```python
from build123d import *

# Parameters (mm, degrees)
BOSS_EXTRUDE1_DEPTH = 1
SKETCH2_W           = 3
SKETCH2_H           = 2.1
SKETCH2_W_2         = 1.6
SKETCH2_H_2         = 0.5
BOSS_EXTRUDE2_DEPTH = 0.1


with BuildPart() as part:
    # Sketch1 → Boss-Extrude1 (new body)
    with BuildSketch(Plane(origin=(0, 0, 0), x_dir=(1, 0, 0), z_dir=(0, 1, 0))):
        with BuildLine():
            Line((-10, 6.5), (10, 6.5))
            Line((10, 6.5), (10, 1))
            Line((10, 1), (9.1, 1))
            ThreePointArc((9.1, 1), (8.1, 0), (9.1, -1))
            Line((9.1, -1), (10, -1))
            Line((10, -1), (10, -6.5))
            Line((10, -6.5), (-10, -6.5))
            Line((-10, -6.5), (-10, -1))
            Line((-10, -1), (-9.1, -1))
            ThreePointArc((-9.1, -1), (-8.1, 0), (-9.1, 1))
            Line((-9.1, 1), (-10, 1))
            Line((-10, 1), (-10, 6.5))
        make_face()
    extrude(amount=BOSS_EXTRUDE1_DEPTH)

    # Sketch2 → Boss-Extrude2 (add)
    with BuildSketch(Plane(origin=(0, 1, 0), x_dir=(1, 0, 0), z_dir=(0, 1, 0))):
        with Locations((-0.175, -5.05)):
            Rectangle(SKETCH2_W, SKETCH2_H)
        with Locations((2.725, -2.5)):
            Rectangle(SKETCH2_W_2, SKETCH2_H_2)
        with Locations((2.725, -1.25)):
            Rectangle(SKETCH2_W_2, SKETCH2_H_2)
        with Locations((2.725, 0)):
            Rectangle(SKETCH2_W_2, SKETCH2_H_2)
        with Locations((2.725, 1.25)):
            Rectangle(SKETCH2_W_2, SKETCH2_H_2)
        with Locations((2.725, 2.5)):
            Rectangle(SKETCH2_W_2, SKETCH2_H_2)
        with Locations((-0.175, 5.05)):
            Rectangle(SKETCH2_W, SKETCH2_H)
    extrude(amount=BOSS_EXTRUDE2_DEPTH)


solid = part.part
```
Could you check a few things on this model? Use its own coordinates, in mm. A direction names the side the tool comes from. Round coordinates to 2 decimals unless told otherwise and drop trailing zeros. Loops run counter-clockwise (first coordinate to the right, second up) from the corner with the lowest first, then second, coordinate; pieces in that order, holes last. Notation, with made-up numbers: M 83,54 L 139,54 A19 cw 139,86 Z; hole C 1.5,53.5 d10. An arc over 180 degrees is marked long. Write item = value, one per line.
1. I need wall thicknesses on probe 1 along Z at (x, y) = (2, 1.05); probe 2 along Y at (x, z) = (0, 3.5). Which ranges of each line are inside material? Lowest first, please.
Results below:
probe_1 = -2.75 to -2.25, -1.5 to -1, -0.25 to 0.25, 1 to 1.5, 2.25 to 2.75
probe_2 = 0 to 1
2. I want a section at A-A, the plane z = 0. Write out the boundary of the cut face in (x, y) (3 decimals).
Results below:
outline = M -8.1,0 L 8.1,0 L 8.1,1 L 3.525,1 L 3.525,1.1 L 1.925,1.1 L 1.925,1 L -8.1,1 Z
3. Will this pin go through, and if not, where does the flat tip stop? P1, Ø2, axis at x = 7.5, z = 2, coming from the +Y side.
Results below:
P1 = 1
4. I want a section at B-B, the plane x = -5.25. Write out the boundary of the cut face in (y, z).
Results below:
outline = M 0,-6.5 L 1,-6.5 L 1,6.5 L 0,6.5 Z
5. I want a section at C-C, the plane z = 5.5. Write out the boundary of the cut face in (x, y) (3 decimals), and give its area (3 significant figures).
Results below:
outline = M -10,0 L 10,0 L 10,1 L 1.325,1 L 1.325,1.1 L -1.675,1.1 L -1.675,1 L -10,1 Z
area = 20.3 mm²
6. I want a section at D-D, the plane z = -3. Write out the boundary of the cut face in (x, y), and give its area (3 significant figures).
Results below:
outline = M -10,0 L 10,0 L 10,1 L -10,1 Z
area = 20.0 mm²
7. Which directions (+Z, -Z, +X, -X, +Y, -Y) give clear straight access to the entire face, cutting with the end or side of a thin tool? Please do faces 1 (the face through (9.5, 0.5, 1)), 2 (the face through (-9.5, 0.5, -1)), 3 (the face through (0.1, 0.5, 6.5)).
Results below:
face_1 = +X, +Y, -Y
face_2 = -X, +Y, -Y
face_3 = +Z, +X, -X, +Y, -Y
